Here's how the part is built. I have some questions about the finished solid (model axes, mm). Face numbers are marked on the shaded views. A direction names the side the tool comes from. Round coordinates to 2 decimals unless told otherwise and drop trailing zeros. Loops run counter-clockwise (first coordinate to the right, second up) from the corner with the lowest first, then second, coordinate; pieces in that order, holes last. Notation, with made-up numbers: (17, 10) - (21, 10) arc R23 ccw to (21, 19) - close; hole circle Ø5 at (-11.5, 12.25). An arc over 180 degrees is marked (long way). Answer as a JSON object with one key per item and string values. Group by question number.
1) I want a section at A-A, the plane z = 26. Please give me the cut outline in (x, y).
2) If we mould it in two halves opening along Z, with no side actions, what happens to the marked faces 1, 2 and 3? For each: pulls with the +Z half, pulls with the -Z half, needs draft (parallel to the pull), parting line crosses it, or undercut.
3) I want a section at B-B, the plane x = -3. Please give me the cut outline in (y, z).
4) I want a section at C-C, the plane x = -45.75. Give the number of separate pieces and of enclosed holes in the cut face, then the cut area to 3 significant figures.
5) Which directions (+Z, -Z, +X, -X, +Y, -Y) give clear straight access to the entire face, cutting with the end or side of a thin tool? Please do the marked faces 4 and 5.
6) If I drill on line 1 along X through (y, z) = (0.25, -31.75); line 2 along Z through (x, y) = (44, -17); line 3 along X through (y, z) = (-14.5, 31.75), over which ranges is the centre line in solid material (lowest first)? Write a range as [from, to].
7) Will these pins go through, and if not, where does the flat tip stop? P1, Ø1.6, axis at y = 1, z = -34.5, coming from the -X side; P2, Ø4, axis at y = -9.5, z = 2, coming from the +X side; P3, Ø6, axis at x = -45.75, z = -31.75, coming from the -Y side.
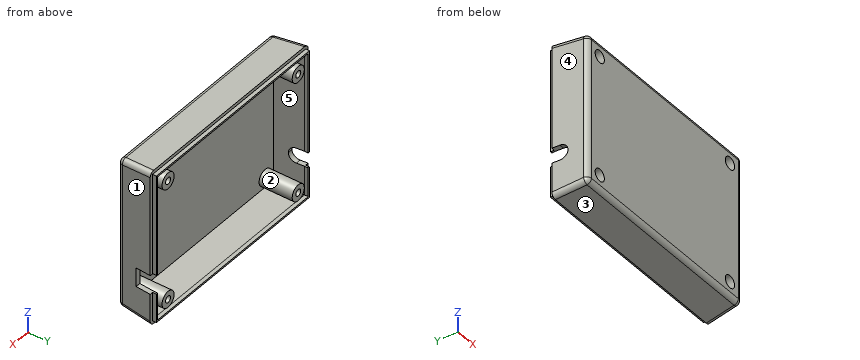
from build123d import *

# Parameters (mm, degrees)
SKETCH_1_W               = 111
SKETCH_1_H               = 82
EXTRUDE_1_DEPTH          = 18
EXTRUDE_1_DRAFT          = -5
SHELL_1_T                = -2.6
FILLET_1_R               = 2.5
SKETCH_2_W               = 107.580136844
SKETCH_2_H               = 78.580136844
SKETCH_2_W_2             = 105.780136844
SKETCH_2_H_2             = 76.780136844
EXTRUDE_2_DEPTH          = 2
SKETCH_4_R               = 4.25
EXTRUDE_3_DEPTH          = 17.5
MIRROR_2_COPY_1_SKETCH_R = 4.25
MIRROR_2_COPY_1_DEPTH    = 17.5
SKETCH_5_R               = 3.25
CUT_EXTRUDE_2_DEPTH      = 17.5
MIRROR_4_COPY_1_SKETCH_R = 3.25
MIRROR_4_COPY_1_DEPTH    = 17.5
SKETCH_6_R               = 1.75
CUT_EXTRUDE_3_DEPTH      = 3
MIRROR_6_COPY_1_SKETCH_R = 1.75
MIRROR_6_COPY_1_DEPTH    = 3
CUT_EXTRUDE_4_DEPTH      = 5
SKETCH_8_W               = 10
SKETCH_8_H               = 10
CUT_EXTRUDE_5_DEPTH      = 5


with BuildPart() as part:
    # Эскиз1 → Бобышка-Вытянуть1 (with draft: the straight prism first)
    with BuildSketch(Plane(origin=(0, 0, 0), x_dir=(1, 0, 0), z_dir=(0, 1, 0))):
        Rectangle(SKETCH_1_W, SKETCH_1_H)
    extrude(amount=-EXTRUDE_1_DEPTH)
    # Бобышка-Вытянуть1: the draft: its side faces are tilted about the plane it starts from
    extrude_1_sides = [part.faces().sort_by_distance(p)[0] for p in [
        (-55.5, -9, 0),
        (0, -9, 41),
        (55.5, -9, 0),
        (0, -9, -41),
    ]]
    draft(extrude_1_sides, Plane(origin=(0, 0, 0), x_dir=(1, 0, 0), z_dir=(0, 1, 0)), EXTRUDE_1_DRAFT)

    # Оболочка1
    shell_1_openings = [part.faces().sort_by_distance(p)[0] for p in [
        (0, 0, 0),
    ]]
    offset(amount=SHELL_1_T, openings=shell_1_openings, kind=Kind.INTERSECTION)

    # Скругление1
    fillet_1_edges = [part.edges().sort_by_distance(p)[0] for p in [
        (53.925204057, -18, 0),
        (0, -18, -39.425204057),
        (-53.925204057, -18, 0),
        (0, -18, 39.425204057),
        (-54.712602028, -9, -40.212602028),
        (54.712602028, -9, -40.212602028),
        (54.712602028, -9, 40.212602028),
        (-54.712602028, -9, 40.212602028),
    ]]
    fillet(fillet_1_edges, radius=FILLET_1_R)

    # Эскиз2 → Бобышка-Вытянуть2 (add)
    with BuildSketch(Plane(origin=(0, 0, 0), x_dir=(1, 0, 0), z_dir=(0, 1, 0))):
        Rectangle(SKETCH_2_W, SKETCH_2_H)
        Rectangle(SKETCH_2_W_2, SKETCH_2_H_2, mode=Mode.SUBTRACT)
    extrude(amount=EXTRUDE_2_DEPTH)

    # Эскиз4 → Бобышка-Вытянуть3 (add)
    with BuildSketch(Plane(origin=(0, -15.4, 0), x_dir=(1, 0, 0), z_dir=(0, 1, 0))):
        with Locations(Location((-45.75, 31.75, 0), (0, 0, 270))):
            Circle(SKETCH_4_R)
    extrude_3 = extrude(amount=EXTRUDE_3_DEPTH)

    # Зеркальное отражение1: Бобышка-Вытянуть3 across plane
    add(extrude_3.mirror(Plane(origin=(0, 0, 0), x_dir=(0, 0, 1), z_dir=(1, 0, 0))))

    # Зеркальное отражение2: Бобышка-Вытянуть3 across plane
    add(extrude_3.mirror(Plane.XY))

    # Зеркальное отражение2 copy 1 sketch → Зеркальное отражение2 copy 1 (add)
    with BuildSketch(Plane(origin=(0, -15.4, 0), x_dir=(-1, 0, 0), z_dir=(0, 1, 0))):
        with Locations(Location((-45.75, 31.75, 0), (0, 0, 270))):
            Circle(MIRROR_2_COPY_1_SKETCH_R)
    extrude(amount=MIRROR_2_COPY_1_DEPTH)

    # Эскиз5 → Вырез-Вытянуть2 (cut)
    with BuildSketch(Plane(origin=(0, -18, 0), x_dir=(1, 0, 0), z_dir=(0, 1, 0))):
        with Locations(Location((-45.75, 31.75, 0), (0, 0, 270))):
            Circle(SKETCH_5_R)
    cut_extrude_2 = extrude(amount=CUT_EXTRUDE_2_DEPTH, mode=Mode.SUBTRACT)

    # Зеркальное отражение3: Вырез-Вытянуть2 across plane
    add(cut_extrude_2.mirror(Plane(origin=(0, 0, 0), x_dir=(0, 0, 1), z_dir=(1, 0, 0))), mode=Mode.SUBTRACT)

    # Зеркальное отражение4: Вырез-Вытянуть2 across plane
    add(cut_extrude_2.mirror(Plane.XY), mode=Mode.SUBTRACT)

    # Зеркальное отражение4 copy 1 sketch → Зеркальное отражение4 copy 1 (cut)
    with BuildSketch(Plane(origin=(0, -18, 0), x_dir=(-1, 0, 0), z_dir=(0, 1, 0))):
        with Locations(Location((-45.75, 31.75, 0), (0, 0, 270))):
            Circle(MIRROR_4_COPY_1_SKETCH_R)
    extrude(amount=MIRROR_4_COPY_1_DEPTH, mode=Mode.SUBTRACT)

    # Эскиз6 → Вырез-Вытянуть3 (cut)
    with BuildSketch(Plane(origin=(0, 2.1, 0), x_dir=(-1, 0, 0), z_dir=(0, 1, 0))):
        with Locations(Location((45.75, -31.75, 0), (0, 0, 90))):
            Circle(SKETCH_6_R)
    cut_extrude_3 = extrude(amount=-CUT_EXTRUDE_3_DEPTH, mode=Mode.SUBTRACT)

    # Зеркальное отражение5: Вырез-Вытянуть3 across plane
    add(cut_extrude_3.mirror(Plane(origin=(0, 0, 0), x_dir=(0, 0, 1), z_dir=(1, 0, 0))), mode=Mode.SUBTRACT)

    # Зеркальное отражение6: Вырез-Вытянуть3 across plane
    add(cut_extrude_3.mirror(Plane.XY), mode=Mode.SUBTRACT)

    # Зеркальное отражение6 copy 1 sketch → Зеркальное отражение6 copy 1 (cut)
    with BuildSketch(Plane(origin=(0, 2.1, 0), x_dir=(1, 0, 0), z_dir=(0, 1, 0))):
        with Locations(Location((45.75, -31.75, 0), (0, 0, 90))):
            Circle(MIRROR_6_COPY_1_SKETCH_R)
    extrude(amount=-MIRROR_6_COPY_1_DEPTH, mode=Mode.SUBTRACT)

    # Эскиз7 → Вырез-Вытянуть4 (cut)
    with BuildSketch(Plane(origin=(-55.5, 0, 0), x_dir=(0, 0, -1), z_dir=(1, 0, 0))):
        with BuildLine():
            Line((19.001, -8), (18.999, -8))
            ThreePointArc((18.999, -8), (16.171279982, -6.828720018), (15, -4.001))
            Line((15, -4.001), (15, 2))
            Line((15, 2), (23, 2))
            Line((23, 2), (23, -4.001))
            ThreePointArc((23, -4.001), (21.828720018, -6.828720018), (19.001, -8))
        make_face()
    extrude(amount=CUT_EXTRUDE_4_DEPTH, mode=Mode.SUBTRACT)

    # Эскиз8 → Вырез-Вытянуть5 (cut)
    with BuildSketch(Plane(origin=(55.5, 0, 0), x_dir=(0, 0, -1), z_dir=(1, 0, 0))):
        with Locations((19, -3)):
            Rectangle(SKETCH_8_W, SKETCH_8_H)
    extrude(amount=-CUT_EXTRUDE_5_DEPTH, mode=Mode.SUBTRACT)


solid = part.part
Outcome:
{
 "1": {"outline": "(-55.5, 0) - (-54.12, -15.72) arc R2.5 ccw to (-51.63, -18) - (51.63, -18) arc R2.5 ccw to (54.12, -15.72) - (55.5, 0) - (53.79, 0) - (53.79, 2) - (52.89, 2) - (52.89, 0) - (51.54, -15.4) - (-51.54, -15.4) - (-52.89, 0) - (-52.89, 2) - (-53.79, 2) - (-53.79, 0) - close"},
 "2": {"face 1": "needs draft", "face 2": "undercut", "face 3": "pulls with the -Z half"},
 "3": {"outline": "(-18, -37.13) arc R2.5 ccw to (-15.72, -39.62) - (0, -41) - (0, -39.29) - (2, -39.29) - (2, -38.39) - (0, -38.39) - (-15.4, -37.04) - (-15.4, 37.04) - (0, 38.39) - (2, 38.39) - (2, 39.29) - (0, 39.29) - (0, 41) - (-15.72, 39.62) arc R2.5 ccw to (-18, 37.13) - close"},
 "4": {"separate pieces": "3", "enclosed holes": "0", "area": "339 mm^2"},
 "5": {"face 4": "+Z, -Z, -X, -Y", "face 5": "+Y"},
 "6": {"line 1": "[-53.79, -52.89], [-50, -47.5], [-44, -41.5], [41.5, 44], [47.5, 50], [52.89, 53.79]", "line 2": "[-39.13, -34.49], [-29.01, 29.01], [34.49, 39.13]", "line 3": "[-54.23, -51.62], [-50, -49], [-42.5, -41.5], [41.5, 42.5], [49, 50], [51.62, 54.23]"},
 "7": {"P1": "x = -53.79", "P2": "x = 54.84", "P3": "y = -0.5"}
}
